```python
from build123d import *

# Parameters (mm, degrees)
SZKIC1_W                    = 8
SZKIC1_H                    = 8
DODANIE_WYCI_GNI_CIE1_DEPTH = 14
SZKIC3_R                    = 1.375
WYTNIJ_WYCI_GNI_CIE1_DEPTH  = 8
WYTNIJ_WYCI_GNI_CIE4_DEPTH  = 4
SZKIC7_W                    = 5
SZKIC7_H                    = 2
WYTNIJ_WYCI_GNI_CIE5_DEPTH  = 5


with BuildPart() as part:
    # Szkic1 → Dodanie-wyciągnięcie1 (new body)
    with BuildSketch(Plane.XY):
        with Locations((4, 4)):
            Rectangle(SZKIC1_W, SZKIC1_H)
    extrude(amount=DODANIE_WYCI_GNI_CIE1_DEPTH)

    # Szkic3 → Wytnij-wyciągnięcie1 (cut)
    with BuildSketch(Plane(origin=(0, 0, 0), x_dir=(-1, 0, 0), z_dir=(0, 0, -1))):
        with Locations((-4, 4)):
            Circle(SZKIC3_R)
    extrude(amount=-WYTNIJ_WYCI_GNI_CIE1_DEPTH, mode=Mode.SUBTRACT)

    # Szkic6 → Wytnij-wyciągnięcie4 (cut)
    with BuildSketch(Plane.XY.offset(14)):
        with BuildLine():
            ThreePointArc((17.051885032, 9.897788808), (8.940279558, 16.987518621), (3, 8))
            Line((3, 8), (8, 8))
            Line((8, 8), (8, 3))
            ThreePointArc((8, 3), (14.233923552, 4.207531496), (17.051885032, 9.897788808))
        make_face()
        with BuildLine():
            Line((8, 8), (3, 8))
            ThreePointArc((3, 8), (4.839078854, 4.839078854), (8, 3))
            Line((8, 3), (8, 8))
        make_face()
    extrude(amount=-WYTNIJ_WYCI_GNI_CIE4_DEPTH, mode=Mode.SUBTRACT)

    # Szkic7 → Wytnij-wyciągnięcie5 (cut)
    with BuildSketch(Plane(origin=(0, 8, 0), x_dir=(1, 0, 0), z_dir=(0, 1, 0))):
        with Locations((5.5, -11)):
            Rectangle(SZKIC7_W, SZKIC7_H)
    extrude(amount=-WYTNIJ_WYCI_GNI_CIE5_DEPTH, mode=Mode.SUBTRACT)


solid = part.part
```
Can you work these out from the model? Positions are in its coordinate system, mm. A direction names the side the tool comes from. Coordinates: 2 decimals unless noted, no trailing zeros. Order: outer loops, then holes, each group sorted by start corner. A loop starts at its lowest first (then second) coordinate and runs counter-clockwise, first axis right, second up.
1. If we section it at B-B (x = 4): Please give me the cut outline in (y, z) (3 decimals), then the cut area to 3 significant figures.
2. If we section it at A-A (z = 4.75): Please give me the cut outline in (x, y) (3 decimals).
3. If we section it at D-D (x = 6.75): Please give me the cut outline in (y, z), then the cut area to 3 significant figures.
4. Thinking about a two-plate mould opening in Z: for faces 1 (the face through (3, 3, 14)), 2 (the face through (5, 3, 11)), 3 (the face through (4, 8, 5)), which applies, +Z half, -Z half, draft (parallel to the pull), parting line (faces both ways), or undercut?
5. For faces 4 (the face through (4.8, 4.88, 13.01)), 5 (the face through (5, 6, 10)), 6 (the face through (2.73, 3.47, 3.94)), 7 (the face through (8, 4, 5)), 8 (the face through (4, 0, 7)), which set-ups out of +Z, -Z, +X, -X, +Y, -Y let a thin tool reach every point of the face, with its end or its side?
6. I need wall thicknesses on line 1 (Z direction, x = 3.25, y = 3.5); line 2 (Y direction, x = 4, z = 6.5) (3 decimals); line 3 (X direction, y = 4.5, z = 0.5). Which ranges of each line are inside material? Lowest first, please.
7. I'm going to push flat-ended pins straight in: pin 1 (2.5 mm diameter, centred on x = 6.5, y = 6.5, fed in from +Z); pin 2 (1.5 mm diameter, centred on x = 5.5, y = 4.5, fed in from -Z); pin 3 (0.8 mm diameter, centred on x = 3.5, y = 4, fed in from -Z). Where does each tip first touch, or does it pass through?
Entries:
1. outline: (0, 0) - (2.625, 0) - (2.625, 8) - (5.375, 8) - (5.375, 0) - (8, 0) - (8, 10) - (3, 10) - (3, 12) - (5.848, 12) - (5.848, 14) - (0, 14) - close
1. area: 75.7 mm2
2. outline: (0, 0) - (8, 0) - (8, 8) - (0, 8) - close; hole circle Ø2.75 at (4, 4)
3. outline: (0, 0) - (8, 0) - (8, 10) - (3, 10) - (3, 12) - (3.47, 12) - (3.47, 14) - (0, 14) - close
3. area: 92.9 mm2
4. face 1: +Z half
4. face 2: undercut
4. face 3: draft
5. face 4: +Z, +X, +Y
5. face 5: +X, +Y
5. face 6: -Z
5. face 7: +Z, -Z, +X, +Y, -Y
5. face 8: +Z, -Z, +X, -X, -Y
6. line 1: z = 8 to 10, 12 to 14
6. line 2: y = 0 to 2.625, 5.375 to 8
6. line 3: x = 0 to 2.72, 5.28 to 8
7. pin 1: stops at z = 10
7. pin 2: stops at z = 0
7. pin 3: stops at z = 8
